from build123d import *

# Parameters (mm, degrees)
F0_R     = 1.625
F1_DEPTH = 4
F2_R     = 4


with BuildPart() as f1:
    # F0 (on Top) → F1 (new body)
    with BuildSketch(Plane.XY):
        Polygon((6, -6), (6, 6), (-6, 6), (-6, -6), (-6, -9), (6, -9), align=None)
        Circle(F0_R, mode=Mode.SUBTRACT)
    extrude(amount=F1_DEPTH)

    # F2
    f2_edges = [f1.edges().sort_by_distance(p)[0] for p in [
        (-6, 6, 2),
        (-6, -9, 2),
        (6, -9, 2),
        (6, 6, 2),
    ]]
    fillet(f2_edges, radius=F2_R)


solid = f1.part
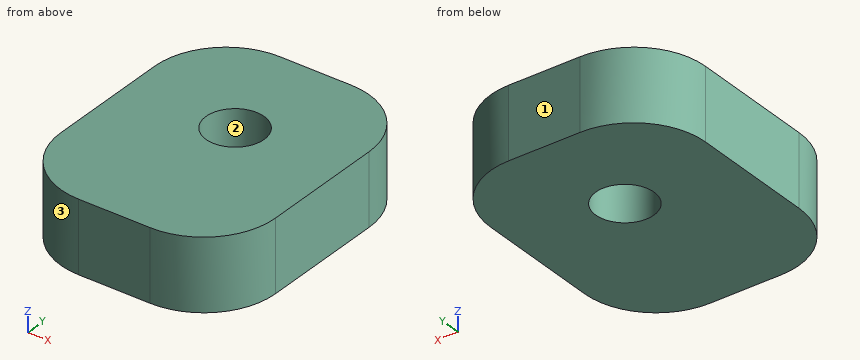
Work out the finished part from the listing and answer in its coordinate system (mm). Face numbers are marked on the shaded views. Coordinates: 2 decimals unless noted, no trailing zeros. Order: outer loops, then holes, each group sorted by start corner. A loop starts at its lowest first (then second) coordinate and runs counter-clockwise, first axis right, second up. Notation, with made-up numbers: (-32, 83) - (-7, 83) arc R27 cw to (-7, 110) - close; hole circle Ø6 at (63.5, -4.75). An arc over 180 degrees is marked (long way). Put each result on its own line as item: value. Start each with the question number.
1) For a pull along X with two mould halves and no side action, classify the marked faces 1, 2 and 3 as released by +X, released by -X, zero draft, split by the parting line, or undercut.
2) Find the intervals of material crossed by line 1 (Y direction, x = 0, z = 2.75) (3 decimals); line 2 (X direction, y = -0.75, z = 3.7); line 3 (Y direction, x = 1.25, z = 3.3), in increasing order. Write a range as from..to.
3) Flat-ended cylindrical pins translate along their axes: pin 1 (2 mm diameter, centred on x = -3.5, z = 2.5, fed in from +Y); pin 2 (2 mm diameter, centred on x = 4, z = 3.5, fed in from -Y); pin 3 (2 mm diameter, centred on x = -3, y = -1.5, fed in from -Z). Find the tip coordinate at first contact, or state that the pin passes through.
4) Find section B-B (x = 0). Give the vertices of the cut face in (y, z) (3 decimals).
5) Find section A-A (z = 3.6). Give the vertices of the cut face in (x, y) (3 decimals).
6) Find section D-D (x = -3.5). Give the vertices of the cut face in (y, z), plus the area to 3 significant figures.
7) Find section C-C (y = 0). Give the vertices of the cut face in (x, z) (3 decimals), plus the area to 3 significant figures.
Results list:
1. face 1: zero draft
1. face 2: undercut
1. face 3: released by -X
2. line 1: y = -9..-1.625, 1.625..6
2. line 2: x = -6..-1.44, 1.44..6
2. line 3: y = -9..-1.04, 1.04..6
3. pin 1: stops at y = 5.97
3. pin 2: stops at y = -8.87
3. pin 3: stops at z = 0
4. outline: (-9, 0) - (-1.625, 0) - (-1.625, 4) - (-9, 4) - close; (1.625, 0) - (6, 0) - (6, 4) - (1.625, 4) - close
5. outline: (-6, -5) arc R4 ccw to (-2, -9) - (2, -9) arc R4 ccw to (6, -5) - (6, 2) arc R4 ccw to (2, 6) - (-2, 6) arc R4 ccw to (-6, 2) - close; hole circle Ø3.25 at (0, 0)
6. outline: (-8.71, 0) - (5.71, 0) - (5.71, 4) - (-8.71, 4) - close
6. area: 57.7 mm^2
7. outline: (-6, 0) - (-1.625, 0) - (-1.625, 4) - (-6, 4) - close; (1.625, 0) - (6, 0) - (6, 4) - (1.625, 4) - close
7. area: 35.0 mm^2
